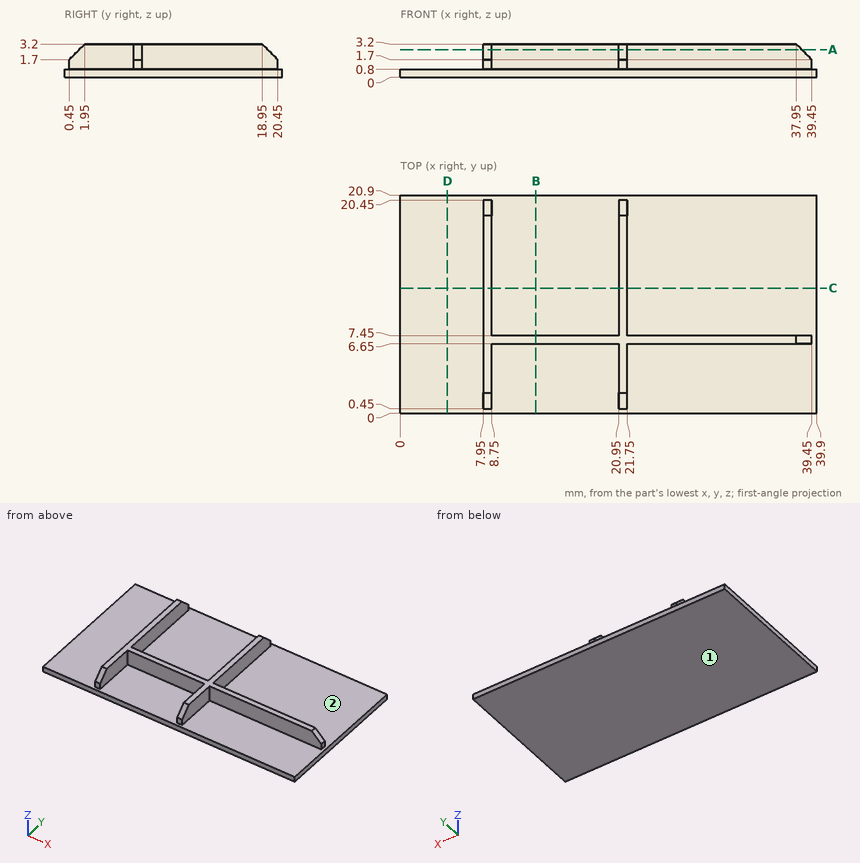
Source: three-view drawing plus pictorial views. Frame: mm from the lowest corner of the part. Give positions to 0.01 mm unless a question says otherwise; leave off trailing zeros. Loops run counter-clockwise (first coordinate to the right, second up) from the corner with the lowest first, then second, coordinate; pieces in that order, holes last. Notation, with made-up numbers: (-7, 24.25) -> (23, 24.25) arc R8 ccw to (23, 28.25) -> close; hole circle Ø6 at (4.25, -31). An arc over 180 degrees is marked (long way). Put each result on its own line as item: value. Start each with the question number.
1) Material intervals for probe 1 along X at (y, z) = (8, 2); probe 2 along Y at (x, z) = (12.5, 2.4); probe 3 along Z at (x, y) = (20, 9), sorted ascending.
2) Draft query along X for the marked faces 1 and 2. Return one class per face: released by +X, released by -X, zero draft, split by the parting line, or undercut.
3) Cut plane B-B (x = 13). Return loops of the section in (y, z), then the cut area to 3 significant figures.
4) Cut plane C-C (y = 12). Return loops of the section in (x, z), then the cut area to 3 significant figures.
5) Contact query for flat-ended pins moving along their axis: P1, Ø0.9, axis at x = 8.5, z = 1.5, coming from the -Y side; P2, Ø1.9, axis at y = 16, z = 2, coming from the +X side; P3, Ø4, axis at x = 11.5, y = 15, coming from the +Z side. Output: stop coordinate, or through.
6) Cut plane A-A (z = 2.65). Return loops of the section in (x, y).
7) Cut plane D-D (x = 4.5). Return loops of the section in (y, z), then the cut area to 3 significant figures.
Results are:
1. probe 1: x = 7.95 to 8.75, 20.95 to 21.75
1. probe 2: y = 6.65 to 7.45
1. probe 3: z = 0 to 0.8
2. face 1: zero draft
2. face 2: undercut
3. outline: (0, 0) -> (20.9, 0) -> (20.9, 0.8) -> (7.45, 0.8) -> (7.45, 3.2) -> (6.65, 3.2) -> (6.65, 0.8) -> (0, 0.8) -> close
3. area: 18.6 mm2
4. outline: (0, 0) -> (39.9, 0) -> (39.9, 0.8) -> (21.75, 0.8) -> (21.75, 3.2) -> (20.95, 3.2) -> (20.95, 0.8) -> (8.75, 0.8) -> (8.75, 3.2) -> (7.95, 3.2) -> (7.95, 0.8) -> (0, 0.8) -> close
4. area: 35.8 mm2
5. P1: stops at y = 0.45
5. P2: stops at x = 21.75
5. P3: stops at z = 0.8
6. outline: (7.95, 1.4) -> (8.75, 1.4) -> (8.75, 6.65) -> (20.95, 6.65) -> (20.95, 1.4) -> (21.75, 1.4) -> (21.75, 6.65) -> (38.5, 6.65) -> (38.5, 7.45) -> (21.75, 7.45) -> (21.75, 19.5) -> (20.95, 19.5) -> (20.95, 7.45) -> (8.75, 7.45) -> (8.75, 19.5) -> (7.95, 19.5) -> close
7. outline: (0, 0) -> (20.9, 0) -> (20.9, 0.8) -> (0, 0.8) -> close
7. area: 16.7 mm2
